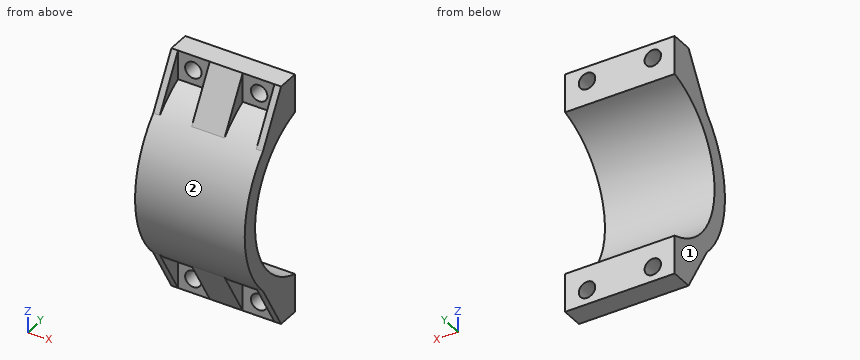
```python
from build123d import *

# Parameters (mm, degrees)
EXTRUDE_1_DEPTH          = 20
RIB_1_REACH              = 37.018
SKETCH_3_WALL_W          = 82.524326188
SKETCH_3_WALL_H          = 1.2
RIB_2_REACH              = 32.434
SKETCH_4_WALL_W          = 73.357332182
SKETCH_4_WALL_H          = 6
MM_1_AT_2_COUNT          = 2
MM_1_AT_2_PITCH          = 12
MIRROR_2_COPY_1_REACH    = 37.018
MIRROR_2_COPY_1_SKETCH_W = 82.524326188
MIRROR_2_COPY_1_SKETCH_H = 1.2


with BuildPart() as part:
    # 草图1 → 凸台-拉伸1 (new body)
    with BuildSketch(Plane(origin=(0, 0, 0), x_dir=(0, 0, -1), z_dir=(1, 0, 0))):
        with BuildLine():
            Line((-22, -4), (-14.974979132, -4))
            ThreePointArc((-14.974979132, -4), (0, -15.5), (14.974979132, -4))
            Line((14.974979132, -4), (22, -4))
            Line((22, -4), (22, -8))
            Line((22, -8), (16.680827318, -8))
            ThreePointArc((16.680827318, -8), (0, -18.5), (-16.680827318, -8))
            Line((-16.680827318, -8), (-22, -8))
            Line((-22, -8), (-22, -4))
        make_face()
    extrude(amount=EXTRUDE_1_DEPTH)

    # 草图3 wall → 筋1 (add, up to next)
    with BuildSketch(Plane(origin=(0, -10.622155252, 17.458293879), x_dir=(0, -0.500000000025, -0.86602540377), z_dir=(0, -0.86602540377, 0.500000000025)), mode=Mode.PRIVATE) as rib_1_sk1:
        with Locations((0, 0.6)):
            Rectangle(SKETCH_3_WALL_W, SKETCH_3_WALL_H)
    rib_1_tool1 = extrude(rib_1_sk1.sketch, amount=-RIB_1_REACH, mode=Mode.PRIVATE) - part.part
    rib_1 = rib_1_tool1.solids().sort_by_distance((0, -10.622155252, 17.458293879))[0]
    add(rib_1)

    # 草图4 wall → 筋2 (add, up to next)
    with BuildSketch(Plane(origin=(10, -10.622155252, 17.458293879), x_dir=(0, -0.500000000025, -0.86602540377), z_dir=(0, -0.86602540377, 0.500000000025)), mode=Mode.PRIVATE) as rib_2_sk1:
        Rectangle(SKETCH_4_WALL_W, SKETCH_4_WALL_H)
    rib_2_tool1 = extrude(rib_2_sk1.sketch, amount=-RIB_2_REACH, mode=Mode.PRIVATE) - part.part
    rib_2 = rib_2_tool1.solids().sort_by_distance((10, -10.622155252, 17.458293879))[0]
    add(rib_2)

    # 镜向1: 筋1 across plane
    add(rib_1.mirror(Plane.ZY.offset(-10)))

    # 草图6 → 大小mm 暗销孔1 (revolve, cut)
    with BuildSketch(Plane(origin=(16, -8, 19.340413659), x_dir=(0, 0, -1), z_dir=(1, 0, 0))):
        Polygon((0, 0), (0, 5.901290929), (1.5, 5), (1.5, 0), align=None)
    mm_1 = revolve(axis=Axis((16, -14.35, 19.340413659), (0, 1, 0)), mode=Mode.SUBTRACT)

    # 大小mm 暗销孔1 at 2: 大小mm 暗销孔1 ×2
    with Locations(*[(-i * MM_1_AT_2_PITCH, 0, 0) for i in range(1, MM_1_AT_2_COUNT)]):
        add(mm_1, mode=Mode.SUBTRACT)

    # 镜向2: 筋1, 筋2, 大小mm 暗销孔1 across plane
    add(rib_1.mirror(Plane.XY))
    add(rib_2.mirror(Plane.XY))
    add(mm_1.mirror(Plane.XY), mode=Mode.SUBTRACT)

    # 镜向2 copy 1 sketch → 镜向2 copy 1 (add, up to next)
    with BuildSketch(Plane(origin=(20, -10.622155252, -17.458293879), x_dir=(0, -0.500000000025, 0.86602540377), z_dir=(0, -0.86602540377, -0.500000000025)), mode=Mode.PRIVATE) as mirror_2_copy_1_sk1:
        with Locations((0, 0.6)):
            Rectangle(MIRROR_2_COPY_1_SKETCH_W, MIRROR_2_COPY_1_SKETCH_H)
    mirror_2_copy_1_tool1 = extrude(mirror_2_copy_1_sk1.sketch, amount=-MIRROR_2_COPY_1_REACH, mode=Mode.PRIVATE) - part.part
    add(mirror_2_copy_1_tool1.solids().sort_by_distance((20, -10.622155252, -17.458293879))[0])

    # 镜向2 copy 2 sketch → 镜向2 copy 2 (revolve, cut)
    with BuildSketch(Plane(origin=(4, -8, -19.340413659), x_dir=(0, 0, 1), z_dir=(1, 0, 0))):
        Polygon((0, 0), (0, -5.901290929), (1.5, -5), (1.5, 0), align=None)
    revolve(axis=Axis((4, -14.35, -19.340413659), (0, -1, 0)), mode=Mode.SUBTRACT)


solid = part.part
```
For this review, take the finished solid that the model builds, in its own axes (mm). Face numbers are marked on the shaded views. A direction names the side the tool comes from. Give positions to 0.01 mm unless a question says otherwise; leave off trailing zeros. Write each loop counter-clockwise with the first axis right and the second up, starting at its lowest first coordinate (ties: lowest second). Pieces come first, ordered by that corner, then holes. Notation, with made-up numbers: M -24.5,85 L 12.5,85 A21 cw 12.5,110 Z; hole C -5.5,18 d9. An arc over 180 degrees is marked long. Answer as a JSON object with one key per item and string values. Group by question number.
Item 1: For probe 1 along Z at (x, y) = (3.5, -5.25); probe 2 along Z at (x, y) = (16, -5.6); probe 3 along Z at (x, y) = (5, -10), list the stretches that pass through material, from the lowest coordinate up. Write a range as [from, to].
Item 2: Consider section C-C on y = -11. Write out the cut boundary in (x, z).
Item 3: Consider section D-D on z = 10.5. Write out the cut boundary in (x, y).
Item 4: Consider section B-B on x = 10.5. Write out the cut boundary in (y, z), plus the area to 3 significant figures.
Item 5: For pin 1 Ø6 at (x, z) = (14.5, -16) entering from -Y; pin 2 Ø3 at (x, z) = (9, 17) entering from -Y; pin 3 Ø5 at (x, z) = (16, 19.34) entering from -Y, all flat-tipped, find the tip position at first contact; note any pin that passes through.
Item 6: Consider section A-A on x = 4. Write out the cut boundary in (y, z), plus the area to 3 significant figures.
Item 7: Tool access review of the marked faces 1 and 2: name each direction out of +Z, -Z, +X, -X, +Y, -Y from which nothing blocks a thin tool from reaching the whole face with its end or side.
Check result:
{
 "1": {"probe 1": "z = [-22, -20.75], [-17.93, -14.58], [14.58, 17.93], [20.75, 22]", "probe 2": "z = [-22, -20.84], [-17.84, -14.45], [14.45, 17.84], [20.84, 22]", "probe 3": "z = [-15.56, -11.84], [11.84, 15.56]"},
 "2": {"outline": "M 0,-16.8 L 1.2,-16.8 L 1.2,-14.87 L 7,-14.87 L 7,-16.8 L 13,-16.8 L 13,-14.87 L 18.8,-14.87 L 18.8,-16.8 L 20,-16.8 L 20,-10.92 L 0,-10.92 Z; M 0,10.92 L 20,10.92 L 20,16.8 L 18.8,16.8 L 18.8,14.87 L 13,14.87 L 13,16.8 L 7,16.8 L 7,14.87 L 1.2,14.87 L 1.2,16.8 L 0,16.8 Z"},
 "3": {"outline": "M 0,-15.23 L 20,-15.23 L 20,-11.4 L 0,-11.4 Z"},
 "4": {"outline": "M -13.24,-12.92 L -8,-22 L -4,-22 L -4,-14.97 A15.5 cw -4,14.97 L -4,22 L -8,22 L -13.24,12.92 A18.5 ccw Z", "area": "198 mm^2"},
 "5": {"pin 1": "stops at y = -13.16", "pin 2": "stops at y = -11.75", "pin 3": "stops at y = -8"},
 "6": {"outline": "M -8,-22 L -4,-22 L -4,-20.84 L -8,-20.84 Z; M -8,-17.84 L -4,-17.84 L -4,-14.97 A15.5 cw -4,14.97 L -4,17.84 L -8,17.84 L -8,16.68 A18.5 ccw -8,-16.68 Z; M -8,20.84 L -4,20.84 L -4,22 L -8,22 Z", "area": "148 mm^2"},
 "7": {"face 1": "+Z, -Z, -X, +Y, -Y", "face 2": "-Y"}
}
